```python
from build123d import *

# Parameters (mm, degrees)
F0_R     = 1.5875
F1_DEPTH = 6


with BuildPart() as f1:
    # F0 (on Top) → F1 (new body)
    with BuildSketch(Plane.XY):
        with BuildLine():
            Line((-109.5, 35), (-109.5, -104.5))
            ThreePointArc((-109.5, -104.5), (-106.413417, -109.119398), (-100.964466, -108.035534))
            Line((-100.964466, -108.035534), (-44.393398, -51.464466))
            ThreePointArc((-44.393398, -51.464466), (-42.771282, -50.380602), (-40.857864, -50))
            Line((-40.857864, -50), (0, -50))
            Line((0, -50), (40.857864, -50))
            ThreePointArc((40.857864, -50), (42.771282, -50.380602), (44.393398, -51.464466))
            Line((44.393398, -51.464466), (100.964466, -108.035534))
            ThreePointArc((100.964466, -108.035534), (106.413417, -109.119398), (109.5, -104.5))
            Line((109.5, -104.5), (109.5, 35))
            ThreePointArc((109.5, 35), (108.336136, 39.556187), (105.129719, 42.995998))
            Line((105.129719, 42.995998), (2.699852, 108.70842))
            ThreePointArc((2.699852, 108.70842), (1.406752, 109.298026), (0, 109.5))
            ThreePointArc((0, 109.5), (-1.406752, 109.298026), (-2.699852, 108.70842))
            Line((-2.699852, 108.70842), (-105.129719, 42.995998))
            ThreePointArc((-105.129719, 42.995998), (-108.336136, 39.556187), (-109.5, 35))
        make_face()
        with Locations((-104.5, -104.5)):
            Circle(F0_R, mode=Mode.SUBTRACT)
        with Locations((-100, -35)):
            Circle(F0_R, mode=Mode.SUBTRACT)
        with Locations((-70, -35)):
            Circle(F0_R, mode=Mode.SUBTRACT)
        with Locations((104.5, -104.5)):
            Circle(F0_R, mode=Mode.SUBTRACT)
        with Locations((0, -20.5)):
            Circle(F0_R, mode=Mode.SUBTRACT)
        with Locations((70, -35)):
            Circle(F0_R, mode=Mode.SUBTRACT)
        with Locations((100, -35)):
            Circle(F0_R, mode=Mode.SUBTRACT)
        with Locations((-100, 35)):
            Circle(F0_R, mode=Mode.SUBTRACT)
        with Locations((-70, 35)):
            Circle(F0_R, mode=Mode.SUBTRACT)
        with Locations((0, 20.5)):
            Circle(F0_R, mode=Mode.SUBTRACT)
        with BuildLine():
            Line((34.255654, 30), (0, 30))
            Line((0, 30), (-34.255654, 30))
            ThreePointArc((-34.255654, 30), (-39.05368, 33.593248), (-36.955506, 39.20842))
            Line((-36.955506, 39.20842), (-2.699852, 61.184647))
            ThreePointArc((-2.699852, 61.184647), (0, 61.976227), (2.699852, 61.184647))
            Line((2.699852, 61.184647), (36.955506, 39.20842))
            ThreePointArc((36.955506, 39.20842), (39.05368, 33.593248), (34.255654, 30))
        make_face(mode=Mode.SUBTRACT)
        with Locations((70, 35)):
            Circle(F0_R, mode=Mode.SUBTRACT)
        with Locations((100, 35)):
            Circle(F0_R, mode=Mode.SUBTRACT)
        with Locations((0, 104.5)):
            Circle(F0_R, mode=Mode.SUBTRACT)
    extrude(amount=F1_DEPTH)


solid = f1.part
```
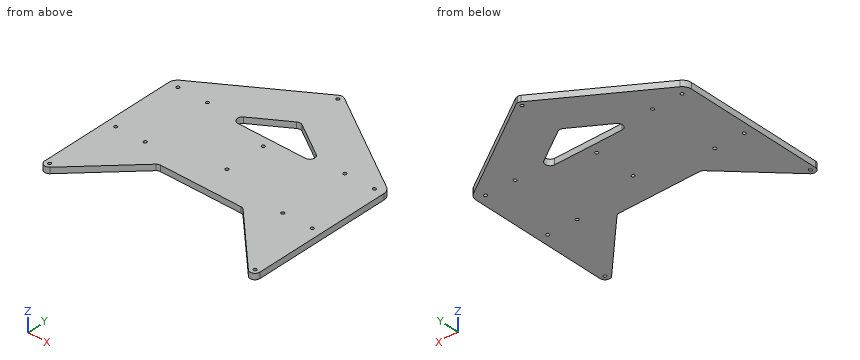
Could you check a few things on this model? Use its own coordinates, in mm. Round coordinates to 2 decimals unless told otherwise and drop trailing zeros. Write each loop counter-clockwise with the first axis right and the second up, starting at its lowest first coordinate (ties: lowest second). Pieces come first, ordered by that corner, then holes. Notation, with made-up numbers: M 58.25,-32.5 L 86.25,-32.5 A22 ccw 86.25,-2.5 Z; hole C -9,39 d5. An arc over 180 degrees is marked long. Answer in a Markdown table with one row per item. Add a question column.
Q1. Imagine slicing it at B-B (y = -77). Please give me the cut outline in (x, z), then the cut area to 3 significant figures.
Q2. Imagine slicing it at C-C (x = 16.5). Please give me the cut outline in (y, z).
Q3. Will these pins go through, and if not, where does the flat tip stop? pin 1 Ø2 at (y, z) = (45.5, 2) entering from +X; pin 2 Ø1.8 at (x, z) = (11, 3) entering from -Y; pin 3 Ø2.5 at (x, y) = (-100, 35) entering from -Z; pin 4 Ø3 at (x, z) = (9.5, 1.5) entering from +Y.
Q4. Imagine slicing it at A-A (z = 1.5). Give the number of separate pieces and of enclosed holes in the cut face, then the cut area to 3 significant figures.
Q5. If I drill on line 1 (Y direction, x = 0, z = 2.85); line 2 (X direction, y = -104.5, z = 1.85); line 3 (Y direction, x = -100, z = 2.8), over which ranges is the centre line in solid material (lowest first)? Write a range as from..to.
Values:
| question | item | result |
|---|---|---|
| 1 | outline | M -109.5,0 L -69.93,0 L -69.93,6 L -109.5,6 Z; M 69.93,0 L 109.5,0 L 109.5,6 L 69.93,6 Z |
| 1 | area | 475 mm^2 |
| 2 | outline | M -50,0 L 30,0 L 30,6 L -50,6 Z; M 52.33,0 L 99.86,0 L 99.86,6 L 52.33,6 Z |
| 3 | pin 1 | x = 102.79 |
| 3 | pin 2 | y = -50 |
| 3 | pin 3 | through |
| 3 | pin 4 | y = 105.31 |
| 4 | separate pieces | 1 |
| 4 | enclosed holes | 14 |
| 4 | area | 30,100 mm^2 |
| 5 | line 1 | -50..-22.09, -18.91..18.91, 22.09..30, 61.98..102.91, 106.09..109.5 |
| 5 | line 2 | -109.5..-106.09, -102.91..-97.43, 97.43..102.91, 106.09..109.5 |
| 5 | line 3 | -107.07..-36.59, -33.41..33.41, 36.59..46.29 |
